Build history of the part. All positions in model axes, mm. A direction names the side the tool comes from. Give positions to 0.01 mm unless a question says otherwise; leave off trailing zeros. Loops run counter-clockwise (first coordinate to the right, second up) from the corner with the lowest first, then second, coordinate; pieces in that order, holes last. Notation, with made-up numbers: M 0,68.25 L 31,68.25 A8 cw 31,82.25 Z; hole C 40.5,43.5 d4. An arc over 180 degrees is marked long. Put each result on its own line as item: value.
Autodesk Inventor part; units mm, degrees
ref_plane "Work Plane1" through (0, 0, 5) normal (0, 0, 1) x (1, 0, 0)
ref_plane "YZ Plane" through (0, 0, 0) normal (1, 0, 0) x (0, 1, 0)
ref_plane "XZ Plane" through (0, 0, 0) normal (0, 1, 0) x (-1, 0, 0)
sketch "Sketch1" plane through (0, 0, 0) normal (0, 0, 1) x (1, 0, 0)
  line L0 (14.6962, 12.74) -> (14.6962, 0) construction
  line L1 (10.61, 12.2) -> (1.53, 12.2)
  arc A0 (1.53, 12.2) -> (0, 10.67) centre (1.53, 10.67) ccw
  line L2 (0, 10.67) -> (0, 1.53)
  arc A1 (0, 1.53) -> (1.53, 0) centre (1.53, 1.53) ccw
  line L3 (1.53, 0) -> (10.61, 0)
  arc A2 (10.61, 0) -> (12.14, 1.53) centre (10.61, 1.53) ccw
  arc A3 (12.14, 10.67) -> (10.61, 12.2) centre (10.61, 10.67) ccw
  line L4 (12.14, 10.67) -> (12.14, 1.53)
  point P0 (0, 0)
  point P1 (0, 0)
  dimension "d10" = 12.74
ref_plane "Work Plane1" through (0, 0, 5) normal (0, 0, 1) x (1, 0, 0)
sketch "Sketch2" plane through (0, 0, 5) normal (0, 0, 1) x (1, 0, 0)
  line L0 (10.88, 12.74) -> (1.8, 12.74)
  line L1 (10.88, 12.74) -> (1.8, 12.74)
  arc A0 (1.8, 12.74) -> (0, 10.94) centre (1.8, 10.94) ccw
  line L2 (0, 10.94) -> (0, 1.8)
  arc A1 (0, 1.8) -> (1.8, 0) centre (1.8, 1.8) ccw
  line L3 (1.8, 0) -> (10.88, 0)
  arc A2 (10.88, 0) -> (12.68, 1.8) centre (10.88, 1.8) ccw
  line L4 (12.68, 1.8) -> (12.68, 10.94)
  arc A3 (12.68, 10.94) -> (10.88, 12.74) centre (10.88, 10.94) ccw
  circle A4 centre (6.34, 6.37) radius 2.8
  line L5 (5.665, 8.395) -> (7.015, 8.395)
  line L6 (7.015, 4.345) -> (5.665, 4.345)
  line L7 (5.665, 4.345) -> (7.015, 8.395) construction
  line L8 (5.665, 8.395) -> (7.015, 4.345) construction
  line L9 (8.365, 5.695) -> (8.365, 7.045)
  line L10 (4.315, 7.045) -> (4.315, 5.695)
  line L11 (4.315, 5.695) -> (8.365, 7.045) construction
  line L12 (8.365, 5.695) -> (4.315, 7.045) construction
  line L13 (4.315, 5.695) -> (5.665, 5.695)
  line L14 (7.015, 5.695) -> (8.365, 5.695)
  line L15 (5.665, 4.345) -> (5.665, 5.695)
  line L16 (5.665, 7.045) -> (5.665, 8.395)
  line L17 (8.365, 7.045) -> (7.015, 7.045)
  line L18 (5.665, 7.045) -> (4.315, 7.045)
  line L19 (7.015, 8.395) -> (7.015, 7.045)
  line L20 (7.015, 5.695) -> (7.015, 4.345)
  point P0 (0, 0)
  dimension "d3" = 5.6
  dimension "d4" = 4.05
  dimension "d5" = 1.35
  dimension "d6" = 4.05
  dimension "d7" = 1.35
extrude "Extrusion3" add sketch "Sketch1" along normal blind 5
sketch "Sketch3" plane through (0, 0, 5) normal (0, 0, 1) x (1, 0, 0)
  line L0 (10.61, 12.47) -> (1.53, 12.47)
  line L1 (10.61, 12.47) -> (1.53, 12.47)
  arc A0 (1.53, 12.47) -> (-0.27, 10.67) centre (1.53, 10.67) ccw
  line L2 (-0.27, 10.67) -> (-0.27, 1.53)
  arc A1 (-0.27, 1.53) -> (1.53, -0.27) centre (1.53, 1.53) ccw
  line L3 (1.53, -0.27) -> (10.61, -0.27)
  arc A2 (10.61, -0.27) -> (12.41, 1.53) centre (10.61, 1.53) ccw
  line L4 (12.41, 1.53) -> (12.41, 10.67)
  arc A3 (12.41, 10.67) -> (10.61, 12.47) centre (10.61, 10.67) ccw
  circle A4 centre (6.07, 6.1) radius 2.8
  line L5 (5.395, 8.125) -> (6.745, 8.125)
  line L6 (6.745, 4.075) -> (5.395, 4.075)
  line L7 (5.395, 4.075) -> (6.745, 8.125) construction
  line L8 (5.395, 8.125) -> (6.745, 4.075) construction
  line L9 (8.095, 5.425) -> (8.095, 6.775)
  line L10 (4.045, 6.775) -> (4.045, 5.425)
  line L11 (4.045, 5.425) -> (8.095, 6.775) construction
  line L12 (8.095, 5.425) -> (4.045, 6.775) construction
  line L13 (4.045, 5.425) -> (5.395, 5.425)
  line L14 (6.745, 5.425) -> (8.095, 5.425)
  line L15 (5.395, 4.075) -> (5.395, 5.425)
  line L16 (5.395, 6.775) -> (5.395, 8.125)
  line L17 (8.095, 6.775) -> (6.745, 6.775)
  line L18 (5.395, 6.775) -> (4.045, 6.775)
  line L19 (6.745, 8.125) -> (6.745, 6.775)
  line L20 (6.745, 5.425) -> (6.745, 4.075)
  line L21 (10.61, 12.2) -> (1.53, 12.2)
  line L22 (0, 10.67) -> (0, 1.53)
  point P0 (0, 0)
  point P1 (-0.27, -0.27)
  point P2 (6.07, 12.2)
  point P3 (0, 6.1)
  point P4 (6.07, 6.1)
  dimension "d14" = 5.6
  dimension "d15" = 4.05
  dimension "d16" = 1.35
  dimension "d17" = 4.05
  dimension "d18" = 1.35
extrude "Extrusion4" add sketch "Sketch3" along normal blind 4.8 contours A4
sketch "Sketch4" plane through (0, 0, 0) normal (0, 0, -1) x (-1, 0, 0)
  line L0 (-13.9436, 0) -> (-13.9436, 2.266)
  line L1 (-15.5559, 0) -> (-15.5559, 6.84)
  line L2 (-1.53, 0) -> (-10.61, 0)
  line L3 (-11.7832, 7.625) -> (-0.3568, 7.625) construction
  line L4 (-0.3568, 7.625) -> (-0.3568, 4.575) construction
  line L5 (-0.3568, 4.575) -> (-11.7832, 4.575) construction
  line L6 (-11.7832, 4.575) -> (-11.7832, 7.625) construction
  line L7 (-11.4668, 4.575) -> (-11.4668, 7.625)
  line L8 (-11.4668, 7.625) -> (-9.4055, 7.625)
  line L9 (-9.4055, 7.625) -> (-9.4055, 7.0442)
  line L10 (-9.4055, 7.0442) -> (-10.7056, 7.0442)
  line L11 (-10.7056, 7.0442) -> (-10.7056, 6.5078)
  line L12 (-10.7056, 6.5078) -> (-9.5068, 6.5078)
  line L13 (-9.5068, 6.5078) -> (-9.5068, 5.927)
  line L14 (-9.5068, 5.927) -> (-10.7056, 5.927)
  line L15 (-10.7056, 5.927) -> (-10.7056, 5.1558)
  line L16 (-10.7056, 5.1558) -> (-9.4055, 5.1558)
  line L17 (-9.4055, 5.1558) -> (-9.4055, 4.575)
  line L18 (-9.4055, 4.575) -> (-11.4668, 4.575)
  line L19 (-6.2739, 4.575) -> (-7.0105, 4.575)
  line L20 (-7.0105, 4.575) -> (-8.187, 6.7006)
  line L21 (-8.187, 6.7006) -> (-8.187, 4.575)
  line L22 (-8.187, 4.575) -> (-8.8864, 4.575)
  line L23 (-8.8864, 4.575) -> (-8.8864, 7.625)
  line L24 (-8.8864, 7.625) -> (-7.9472, 7.625)
  line L25 (-7.9472, 7.625) -> (-6.9734, 5.8776)
  line L26 (-6.9734, 5.8776) -> (-6.9734, 7.625)
  line L27 (-6.9734, 7.625) -> (-6.2739, 7.625)
  line L28 (-6.2739, 7.625) -> (-6.2739, 4.575)
  line L29 (-5.0678, 4.575) -> (-5.0678, 7.0442)
  line L30 (-5.0678, 7.0442) -> (-5.9699, 7.0442)
  line L31 (-5.9699, 7.0442) -> (-5.9699, 7.625)
  line L32 (-5.9699, 7.625) -> (-3.3994, 7.625)
  line L33 (-3.3994, 7.625) -> (-3.3994, 7.0442)
  line L34 (-3.3994, 7.0442) -> (-4.3015, 7.0442)
  line L35 (-4.3015, 7.0442) -> (-4.3015, 4.575)
  line L36 (-4.3015, 4.575) -> (-5.0678, 4.575)
  line L37 (-0.2678, 4.575) -> (-1.1996, 4.575)
  line L38 (-1.1996, 4.575) -> (-2.0474, 5.6947)
  line L39 (-2.0474, 5.6947) -> (-2.3242, 5.6947)
  line L40 (-2.3242, 5.6947) -> (-2.3242, 4.575)
  line L41 (-2.3242, 4.575) -> (-3.0855, 4.575)
  line L42 (-3.0855, 4.575) -> (-3.0855, 7.625)
  line L43 (-3.0855, 7.625) -> (-1.8596, 7.625)
  spline S0 degree 2 poles (-1.8596, 7.625) (-1.605, 7.625) (-1.2293, 7.5607) (-1.0686, 7.4619) knots 0 0 0 1 2 2 2
  spline S1 degree 2 poles (-1.0686, 7.4619) (-0.9055, 7.3581) (-0.7127, 7.0343) (-0.7127, 6.7871) knots 0 0 0 1 2 2 2
  spline S2 degree 2 poles (-0.7127, 6.7871) (-0.7127, 6.4386) (-1.0291, 6.0011) (-1.2936, 5.8726) knots 0 0 0 1 2 2 2
  line L44 (-1.2936, 5.8726) -> (-0.2678, 4.575)
  spline S3 degree 2 poles (-1.4987, 6.6907) (-1.4987, 6.8069) (-1.5877, 6.9725) (-1.689, 7.017) knots 0 0 0 1 2 2 2
  spline S4 degree 2 poles (-1.689, 7.017) (-1.7607, 7.0466) (-1.9362, 7.0639) (-2.0672, 7.0639) knots 0 0 0 1 2 2 2
  line L45 (-2.0672, 7.0639) -> (-2.3242, 7.0639)
  line L46 (-2.3242, 7.0639) -> (-2.3242, 6.2434)
  line L47 (-2.3242, 6.2434) -> (-2.1043, 6.2434)
  spline S5 degree 2 poles (-2.1043, 6.2434) (-1.9461, 6.2434) (-1.7212, 6.2829) (-1.6445, 6.3447) knots 0 0 0 1 2 2 2
  spline S6 degree 2 poles (-1.6445, 6.3447) (-1.5704, 6.404) (-1.4987, 6.5622) (-1.4987, 6.6907) knots 0 0 0 1 2 2 2
  point P0 (0, 0)
  point P1 (-6.07, 0)
  point P2 (-6.07, 2.266)
  point P3 (-6.07, 6.84)
  point P4 (-6.07, 6.1)
  point P5 (-6.07, 4.575)
  point P6 (-0.3568, 6.1)
  point P7 (-6.07, 6.1)
  dimension "d21" = 2.266
  dimension "d22" = 6.84
extrude "Extrusion5" add sketch "Sketch4" along normal blind 0.9
properties part number "IPC ENTR key"
Q1. Slice it at C-C (y = 1.75). List the corners of the cut face in (x, z), and give its area (3 significant figures).
Here are the results:
outline: M 0,0 L 12.14,0 L 12.14,5 L 0,5 Z
area: 60.7 mm²
Q2. Slice it at B-B (x = 10). List the corners of the cut face in (y, z) (3 decimals), and give its area (3 significant figures).
Here are the results:
outline: M 0,0 L 4.575,0 L 4.575,-0.9 L 5.156,-0.9 L 5.156,0 L 5.927,0 L 5.927,-0.9 L 6.508,-0.9 L 6.508,0 L 7.044,0 L 7.044,-0.9 L 7.625,-0.9 L 7.625,0 L 12.2,0 L 12.2,5 L 0,5 Z
area: 62.6 mm²
Q3. Slice it at A-A (z = 6.25). List the corners of the cut face in (x, y) (3 decimals).
Here are the results:
outline: C 6.07,6.1 d5.6; hole M 4.045,5.425 L 5.395,5.425 L 5.395,4.075 L 6.745,4.075 L 6.745,5.425 L 8.095,5.425 L 8.095,6.775 L 6.745,6.775 L 6.745,8.125 L 5.395,8.125 L 5.395,6.775 L 4.045,6.775 Z
Q4. Tool access for faces 4 (the flat face through (10.4, 4.575, -0.4)), 5 (the flat face through (10.1, 6.508, -0.4)), 6 (the flat face through (0.788, 5.233, -0.444)), 7 (the flat face through (8.886, 6.1, -0.4)): list every direction of +Z, -Z, +X, -X, +Y, -Y with a clear straight run to the whole face (end or side of a thin tool).
Here are the results:
face 4: -Z, +X, -X, -Y
face 5: -Z
face 6: -Z, -X
face 7: -Z, +Y, -Y
Q5. Mould opens along Y. For faces 1 (the flat face through (2.5, 7.625, -0.4)), 2 (the flat face through (6.745, 7, 7)), 3 (the flat face through (7.6, 6.1, -0.9)) say: pulls with the +Y half, pulls with the -Y half, needs draft (parallel to the pull), parting line crosses it, or undercut.
Here are the results:
face 1: pulls with the +Y half
face 2: undercut
face 3: needs draft
Q6. Slice it at D-D (x = 7.25). List the corners of the cut face in (y, z) (3 decimals), and give its area (3 significant figures).
Here are the results:
outline: M 0,0 L 5.008,0 L 5.008,-0.9 L 6.374,-0.9 L 6.374,0 L 12.2,0 L 12.2,5 L 8.639,5 L 8.639,9.8 L 6.775,9.8 L 6.775,5 L 5.425,5 L 5.425,9.8 L 3.561,9.8 L 3.561,5 L 0,5 Z
area: 80.1 mm²
Q7. Probe line 1 (Y direction, x = 6, z = 5.75) (3 decimals); line 2 (Z direction, x = 2.75, y = 5); line 3 (X direction, y = 6.25, z = 7.75) (3 decimals). List the from-to ranges inside material, lowest first. Write a range as from..to.
Here are the results:
line 1: 3.301..4.075, 8.125..8.899
line 2: -0.9..5
line 3: 3.274..4.045, 8.095..8.866
Q8. Drop flat-ended pins along their axis: pin 1 Ø4 at (x, z) = (9, 7.5) entering from +Y; pin 2 Ø6 at (x, y) = (6, 4) entering from -Z; pin 3 Ø1.5 at (x, z) = (4.5, 6.5) entering from +Y; pin 4 Ø0.8 at (x, z) = (8.5, -0.5) entering from -Y (3 decimals). Give the stop position or say it passes through.
Here are the results:
pin 1: y = 8.74
pin 2: z = -0.9
pin 3: y = 8.78
pin 4: y = 4.575
